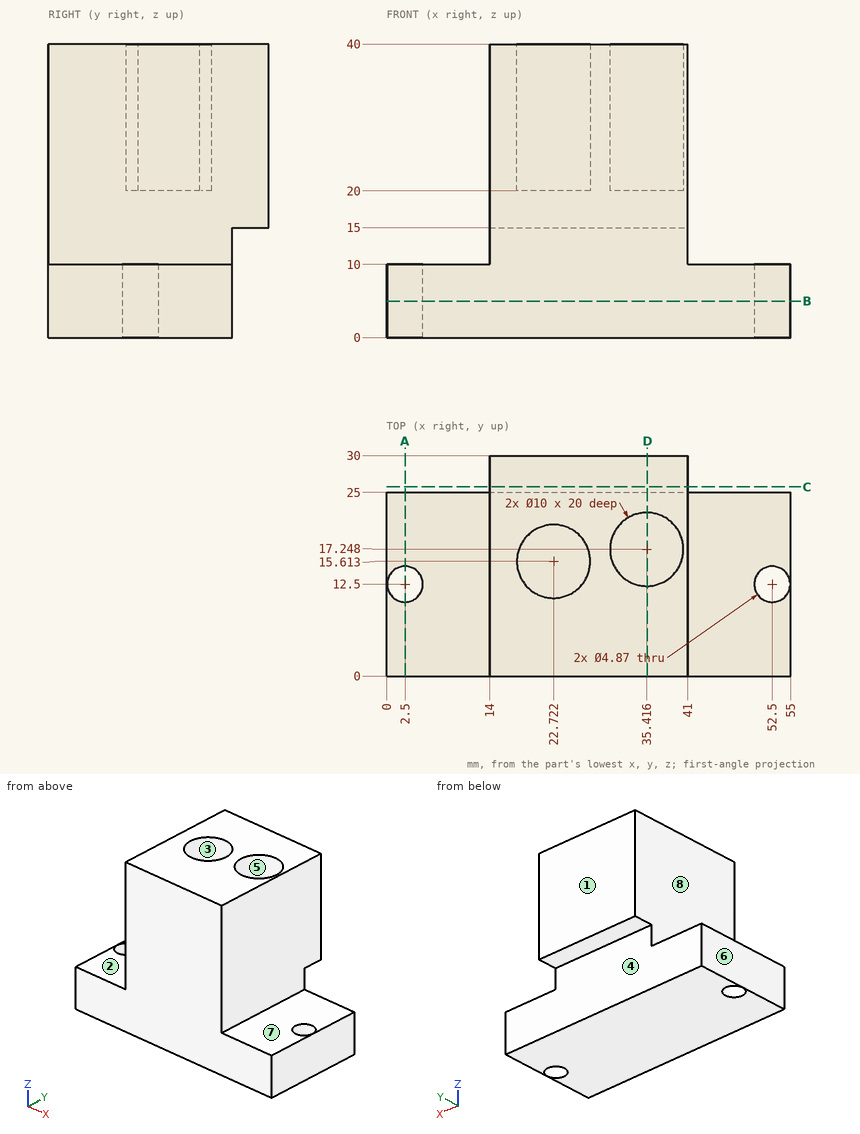
Study the drawing (mm; zero at the part's minimum x, y, z) and answer. A direction names the side the tool comes from. Give positions to 0.01 mm unless a question says otherwise; leave off trailing zeros. Order: outer loops, then holes, each group sorted by start corner. A loop starts at its lowest first (then second) coordinate and runs counter-clockwise, first axis right, second up. Notation, with made-up numbers: (71.25, -18.5) -> (90.25, -18.5) arc R33 ccw to (90.25, 11.5) -> close; hole circle Ø11 at (-7.5, 19). An arc over 180 degrees is marked (long way). Put each result on its own line as item: value.
Item 1: For a pull along Y with two mould halves and no side action, classify the marked faces 1, 2 and 3 as released by +Y, released by -Y, zero draft, split by the parting line, or undercut.
Established:
face 1: released by +Y
face 2: zero draft
face 3: undercut
Item 2: A cutting plane is placed at B-B on z = 5. Give the vertices of the cut face in (x, y) (1 decimal), plus the area to 3 significant figures.
Established:
outline: (0, 0) -> (55, 0) -> (55, 25) -> (0, 25) -> close; hole circle Ø4.9 at (2.5, 12.5); hole circle Ø4.9 at (52.5, 12.5)
area: 1,340 mm^2
Item 3: A cutting plane is placed at C-C on y = 25.75. Give the vertices of the cut face in (x, z).
Established:
outline: (14, 15) -> (41, 15) -> (41, 40) -> (14, 40) -> close
Item 4: For the marked faces 4, 5, 6, 7 and 8, determine the directions among +Z, -Z, +X, -X, +Y, -Y from which every point of the face is accessible in a straight line to the end or side of a thin tool.
Established:
face 4: -Z, +X, -X, +Y
face 5: +Z
face 6: +Z, -Z, -X, +Y, -Y
face 7: +Z, +X, +Y, -Y
face 8: +Z, -X, +Y, -Y
Item 5: A cutting plane is placed at D-D on x = 35.5. Give the vertices of the cut face in (y, z), plus the area to 3 significant figures.
Established:
outline: (0, 0) -> (25, 0) -> (25, 15) -> (30, 15) -> (30, 40) -> (22.25, 40) -> (22.25, 20) -> (12.25, 20) -> (12.25, 40) -> (0, 40) -> close
area: 925 mm^2
Item 6: A cutting plane is placed at A-A on x = 2.5. Give the vertices of the cut face in (y, z) (1 decimal), plus the area to 3 significant figures.
Established:
outline: (0, 0) -> (10.1, 0) -> (10.1, 10) -> (0, 10) -> close; (14.9, 0) -> (25, 0) -> (25, 10) -> (14.9, 10) -> close
area: 201 mm^2
Item 7: Straight lines are drawn through the part: line 1 (Y direction, x = 52.5, z = 2.5) (1 decimal); line 2 (X direction, y = 16.75, z = 34.5); line 3 (Y direction, x = 37, z = 5). For each, find the intervals that lie inside material, in ascending order.
Established:
line 1: y = 0 to 10.1, 14.9 to 25
line 2: x = 14 to 17.85, 27.59 to 30.44, 40.39 to 41
line 3: y = 0 to 25
Item 8: Given P1, Ø1.5, axis at x = 49, z = 5, coming from the +Y side; P2, Ø10, axis at y = 13, z = 26, coming from the -X side; P3, Ø4, axis at x = 52.5, y = 12.5, coming from the -Z side; P4, Ø5, axis at x = 34, y = 16, coming from the +Z side, each flat-ended and moving along its own axis, determine where each tip first touches the part or whether it passes through.
Established:
P1: stops at y = 25
P2: stops at x = 14
P3: passes through
P4: stops at z = 20
